Can you work these out from the model? Positions are in its coordinate system, mm. Face numbers are marked on the shaded views. Round coordinates to 2 decimals unless told otherwise and drop trailing zeros. Order: outer loops, then holes, each group sorted by start corner. A loop starts at its lowest first (then second) coordinate and runs counter-clockwise, first axis right, second up.
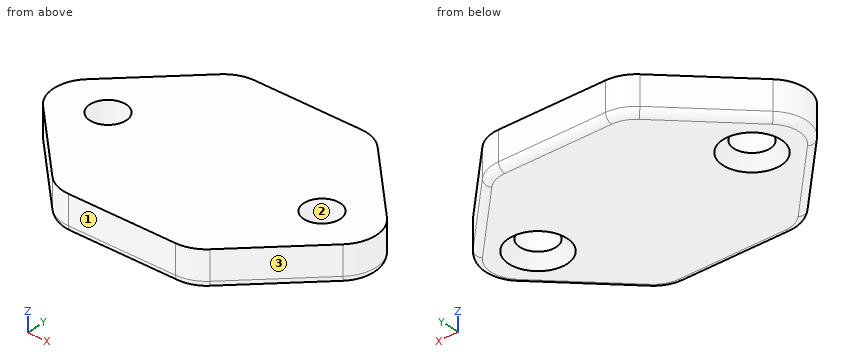
from build123d import *

# Parameters (mm, degrees)
SKETCH_R         = 2.5
PAD_DEPTH        = 5
FILLET_R         = 5
FILLET001_R      = 1
HOLE_D           = 5
HOLE_CSINK_D     = 8
HOLE_CSINK_ANGLE = 90


with BuildPart() as part:
    # Sketch → Pad (new body)
    with BuildSketch(Plane.XY):
        with BuildLine():
            Line((-21.035534, 3.535534), (-9.571068, 15))
            Line((-9.571068, 15), (9.571068, 15))
            Line((9.571068, 15), (21.035534, 3.535534))
            ThreePointArc((21.035534, -3.535534), (22.5, 0), (21.035534, 3.535534))
            Line((21.035534, -3.535534), (9.571068, -15))
            Line((9.571068, -15), (-9.571068, -15))
            Line((-9.571068, -15), (-21.035534, -3.535534))
            ThreePointArc((-21.035534, 3.535534), (-22.5, 0), (-21.035534, -3.535534))
        make_face()
        with Locations((-15, 0)):
            Circle(SKETCH_R, mode=Mode.SUBTRACT)
        with Locations((15, 0)):
            Circle(SKETCH_R, mode=Mode.SUBTRACT)
    extrude(amount=PAD_DEPTH)

    # Fillet
    fillet_edges = [part.edges().sort_by_distance(p)[0] for p in [
        (9.571068, -15, 2.5),
        (-9.571068, -15, 2.5),
        (9.571068, 15, 2.5),
        (-9.571068, 15, 2.5),
    ]]
    fillet(fillet_edges, radius=FILLET_R)

    # Fillet001
    fillet001_edges = [part.edges().sort_by_distance(p)[0] for p in [
        (-16.035534, 8.535534, 0),
        (-9.413417, 14.619398, 0),
        (-22.5, 0, 0),
        (0, 15, 0),
        (-16.035534, -8.535534, 0),
        (9.413417, 14.619398, 0),
        (-9.413417, -14.619398, 0),
        (16.035534, 8.535534, 0),
        (0, -15, 0),
        (22.5, 0, 0),
        (9.413417, -14.619398, 0),
        (16.035534, -8.535534, 0),
        (12.5, 0, 0),
        (-17.5, 0, 0),
    ]]
    fillet(fillet001_edges, radius=FILLET001_R)

    # Hole (through all)
    with Locations(Plane(origin=(0, 0, 0), x_dir=(1, 0, 0), z_dir=(0, 0, -1))):
        with Locations((-15, 0), (15, 0)):
            CounterSinkHole(HOLE_D / 2, HOLE_CSINK_D / 2, counter_sink_angle=HOLE_CSINK_ANGLE)


solid = part.part
(1) Please list where these lines run through material, in increasing order: probe 1 along X at (y, z) = (0, 2.45); probe 2 along X at (y, z) = (-2.25, 4.5); probe 3 along Y at (x, z) = (10.5, 2.2).
(2) I want a section at A-A, the plane y = 0. List the corners of the cut face in (x, z) for me, plus the area to 3 significant figures.
(3) I want a section at B-B, the plane z = 4.35. List the corners of the cut face in (x, y) for me, plus the area to 3 significant figures.
(4) I'm going to push flat-ended pins straight in: pin 1 Ø1.5 at (x, y) = (4, -7.5) entering from -Z; pin 2 Ø1 at (x, z) = (-8.5, 2.5) entering from +Y. Where does each tip first touch, or does it pass through?
(5) If we mould it in two halves opening along X, with no side actions, what happens to the marked faces 1, 2 and 3? For each: pulls with the +X half, pulls with the -X half, needs draft (parallel to the pull), parting line crosses it, or undercut.
Ans:
1. probe 1: x = -22.5 to -17.5, -12.5 to 12.5, 17.5 to 22.5
1. probe 2: x = -21.97 to -16.09, -13.91 to 13.91, 16.09 to 21.97
1. probe 3: y = -14 to 14
2. outline: (-22.5, 1) arc R1 ccw to (-21.5, 0) - (-19, 0) - (-17.5, 1.5) - (-17.5, 5) - (-22.5, 5) - close; (-12.5, 1.5) - (-11, 0) - (11, 0) - (12.5, 1.5) - (12.5, 5) - (-12.5, 5) - close; (17.5, 1.5) - (19, 0) - (21.5, 0) arc R1 ccw to (22.5, 1) - (22.5, 5) - (17.5, 5) - close
2. area: 170 mm2
3. outline: (-21.04, -3.54) - (-11.04, -13.54) arc R5 ccw to (-7.5, -15) - (7.5, -15) arc R5 ccw to (11.04, -13.54) - (21.04, -3.54) arc R5 ccw to (21.04, 3.54) - (11.04, 13.54) arc R5 ccw to (7.5, 15) - (-7.5, 15) arc R5 ccw to (-11.04, 13.54) - (-21.04, 3.54) arc R5 ccw to start; hole circle Ø5 at (-15, 0); hole circle Ø5 at (15, 0)
3. area: 972 mm2
4. pin 1: stops at z = 0
4. pin 2: stops at y = 14.97
5. face 1: needs draft
5. face 2: undercut
5. face 3: pulls with the +X half
